Model file for the job. Use its own axes, mm. Face numbers are marked on the shaded views. A direction names the side the tool comes from. Round coordinates to 2 decimals unless told otherwise and drop trailing zeros. Order: outer loops, then holes, each group sorted by start corner. A loop starts at its lowest first (then second) coordinate and runs counter-clockwise, first axis right, second up. Notation, with made-up numbers: (25.25, 3.5) -> (42.25, 3.5) arc R37 ccw to (42.25, 42.5) -> close; hole circle Ø1 at (79.25, -35). An arc over 180 degrees is marked (long way). Answer as CSV lines item,"result".
```python
from build123d import *
from OCP.BRepFilletAPI import BRepFilletAPI_MakeChamfer

# Parameters (mm, degrees)
BOSS_EXTRU_1_DEPTH      = 75
ESQUISSE2_W             = 11.9
ESQUISSE2_H             = 4
ENL_V_MAT_EXTRU_1_DEPTH = 10
BOSS_EXTRU_2_START      = 0.5
BOSS_EXTRU_2_DEPTH      = 3
ESQUISSE4_W             = 3
ESQUISSE4_H             = 8
BOSS_EXTRU_3_DEPTH      = 2
ESQUISSE5_W             = 11.9
ESQUISSE5_H             = 1.2
ENL_V_MAT_EXTRU_2_DEPTH = 3
CHANFREIN1_SIZE         = 0.5
CONG_1_R                = 0.25
BOSS_EXTRU_4_DEPTH      = 0.1
CHANFREIN2_SIZE         = 0.3
CHANFREIN2_SIZE_2       = 2.134610917
CHANFREIN3_SIZE         = 0.3
CHANFREIN3_SIZE_2       = 2.134610917


with BuildPart() as part:
    # Esquisse1 → Boss.-Extru.1 (new body)
    with BuildSketch(Plane(origin=(0, 0, 0), x_dir=(0, 0, -1), z_dir=(1, 0, 0))):
        Polygon((0, 0), (0, 2.6), (8, 2.6), (8, 4.65), (19.6, 4.65), (19.6, 8.2), (22.6, 8.2), (22.6, 1.2), (2.6, 1.2), (2.6, 0), align=None)
    extrude(amount=BOSS_EXTRU_1_DEPTH)

    # Esquisse2 → Enlèv. mat.-Extru.1 (cut)
    with BuildSketch(Plane(origin=(0, 2.6, 0), x_dir=(1, 0, 0), z_dir=(0, 1, 0))):
        with Locations((10.95, 5)):
            Rectangle(ESQUISSE2_W, ESQUISSE2_H)
    extrude(amount=-ENL_V_MAT_EXTRU_1_DEPTH, mode=Mode.SUBTRACT)

    # Esquisse3 → Boss.-Extru.2 (add)
    with BuildSketch(Plane.XY.offset(-7).offset(BOSS_EXTRU_2_START)):
        Polygon((5, 2.6), (11.9, 2.3), (11.9, 0.9), (5, 1.2), align=None)
    extrude(amount=BOSS_EXTRU_2_DEPTH)

    # Esquisse4 → Boss.-Extru.3 (add)
    with BuildSketch(Plane(origin=(0, 2.6, 0), x_dir=(1, 0, 0), z_dir=(0, 1, 0))):
        with Locations((73.5, 4)):
            Rectangle(ESQUISSE4_W, ESQUISSE4_H)
    extrude(amount=BOSS_EXTRU_3_DEPTH)

    # Esquisse5 → Enlèv. mat.-Extru.2 (cut)
    with BuildSketch(Plane.XY):
        with Locations((5.95, 0.6)):
            Rectangle(ESQUISSE5_W, ESQUISSE5_H)
    extrude(amount=-ENL_V_MAT_EXTRU_2_DEPTH, mode=Mode.SUBTRACT)

    # Chanfrein1
    chanfrein1_edges = [part.edges().sort_by_distance(p)[0] for p in [
        (0, 2.6, -4),
        (0, 6.425, -19.6),
        (0, 1.2, -11.3),
        (11.9, 0, -1.3),
    ]]
    chamfer(chanfrein1_edges, length=CHANFREIN1_SIZE)

    # Congé1
    cong_1_edges = [part.edges().sort_by_distance(p)[0] for p in [
        (5, 1.9, -7),
        (5, 1.9, -3),
        (5, 1.9, -6.5),
        (5, 1.9, -3.5),
    ]]
    fillet(cong_1_edges, radius=CONG_1_R - 0.0001)  # a hair under: the kernel refuses the full size

    # Esquisse6 → Boss.-Extru.4 (add, symmetric)
    with BuildSketch(Plane(origin=(37.5, 0, 0), x_dir=(0, 0, -1), z_dir=(1, 0, 0))):
        Polygon((0, 0), (0, -0.3), (2.9, -0.3), (2.9, 1.2), (2.6, 1.2), (2.6, 0), align=None)
    extrude(amount=BOSS_EXTRU_4_DEPTH, both=True)

    # Chanfrein2
    chanfrein2_edges_1 = [part.edges().sort_by_distance(p)[0] for p in [
        (37.4, 0.6, -2.6),
    ]]
    chanfrein2_side_1 = [part.faces().sort_by_distance(p)[0] for p in [
        (37.4, 0.6, -2.606),
    ]]
    chanfrein2_edges_2 = [part.edges().sort_by_distance(p)[0] for p in [
        (37.4, 0, -1.3),
    ]]
    chanfrein2_side_2 = [part.faces().sort_by_distance(p)[0] for p in [
        (37.394, 0, -1.3),
    ]]
    chanfrein2 = BRepFilletAPI_MakeChamfer(part.part.solid().wrapped)
    for e in chanfrein2_edges_1:
        chanfrein2.Add(CHANFREIN2_SIZE - 0.0001, CHANFREIN2_SIZE_2 - 0.0001, e.wrapped, chanfrein2_side_1[0].wrapped)
    for e in chanfrein2_edges_2:
        chanfrein2.Add(CHANFREIN2_SIZE_2 - 0.0001, CHANFREIN2_SIZE - 0.0001, e.wrapped, chanfrein2_side_2[0].wrapped)
    add(Compound.cast(chanfrein2.Shape()), mode=Mode.REPLACE)  # a hair under: the kernel refuses the full size

    # Chanfrein3
    chanfrein3_edges_1 = [part.edges().sort_by_distance(p)[0] for p in [
        (37.6, 0.6, -2.6),
    ]]
    chanfrein3_side_1 = [part.faces().sort_by_distance(p)[0] for p in [
        (37.6, 0.6, -2.606),
    ]]
    chanfrein3_edges_2 = [part.edges().sort_by_distance(p)[0] for p in [
        (37.6, 0, -1.3),
    ]]
    chanfrein3_side_2 = [part.faces().sort_by_distance(p)[0] for p in [
        (37.6, -0.006, -1.3),
    ]]
    chanfrein3 = BRepFilletAPI_MakeChamfer(part.part.solid().wrapped)
    for e in chanfrein3_edges_1:
        chanfrein3.Add(CHANFREIN3_SIZE - 0.0001, CHANFREIN3_SIZE_2 - 0.0001, e.wrapped, chanfrein3_side_1[0].wrapped)
    for e in chanfrein3_edges_2:
        chanfrein3.Add(CHANFREIN3_SIZE - 0.0001, CHANFREIN3_SIZE_2 - 0.0001, e.wrapped, chanfrein3_side_2[0].wrapped)
    add(Compound.cast(chanfrein3.Shape()), mode=Mode.REPLACE)  # a hair under: the kernel refuses the full size


solid = part.part
```
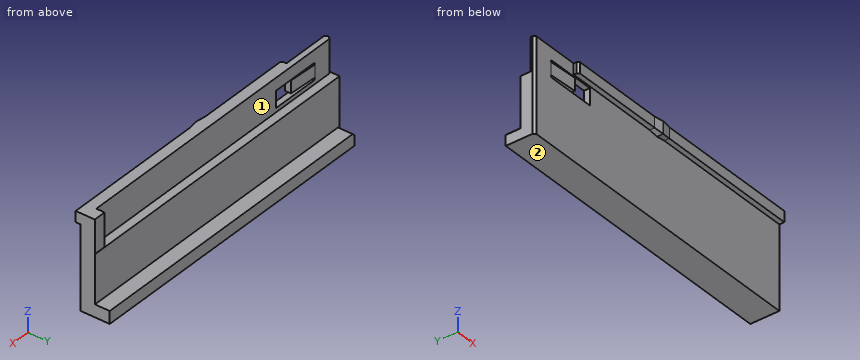
Q1. Saw through at C-C (x = 46). Write the cut outline in (y, z), plus the area to 3 significant figures.
Checks:
outline,"(0, -2.6) -> (1.2, -2.6) -> (1.2, -22.6) -> (8.2, -22.6) -> (8.2, -19.6) -> (4.65, -19.6) -> (4.65, -8) -> (2.6, -8) -> (2.6, 0) -> (0, 0) -> close"
area,"75.3 mm²"
Q2. Saw through at B-B (y = 3.75). Write the cut outline in (x, z).
Checks:
outline,"(0, -22.6) -> (75, -22.6) -> (75, 0) -> (72, 0) -> (72, -8) -> (0, -8) -> close"
Q3. Tool access for the marked faces 1 and 2: list every direction of +Z, -Z, +X, -X, +Y, -Y with a clear straight run to the whole face (end or side of a thin tool).
Checks:
face 1,"+Z, -X, +Y"
face 2,"-Z, +X, -X, +Y, -Y"
Q4. Wall check: L1, parallel to Y at x = 37.5, z = -12.5; L2, parallel to Z at x = 23, y = 4.5; L3, parallel to Y at x = 36, z = -7.25. Give the ranges that are in metal, low to high. Write a range as [from, to].
Checks:
L1,"[1.2, 4.65]"
L2,"[-22.6, -8]"
L3,"[1.2, 2.6]"
Q5. Saw through at D-D (z = -14.75). Write the cut outline in (x, y), plus the area to 3 significant figures.
Checks:
outline,"(0, 1.7) -> (0.5, 1.2) -> (75, 1.2) -> (75, 4.65) -> (0, 4.65) -> close"
area,"259 mm²"
Q6. Flat gauge pins, fed straight in: pin 1 (1 mm diameter, centred on x = 39, z = -6.5, fed in from +Y); pin 2 (4 mm diameter, centred on x = 39, y = 6.5, fed in from +Z); pin 3 (1.3 mm diameter, centred on x = 20, z = -0.5, fed in from -Y). Where does each tip first touch, or does it go through?
Checks:
pin 1,"y = 2.6"
pin 2,"z = -8"
pin 3,"y = 0"
